Autodesk Inventor part; units mm, degrees
ref_plane "YZ Plane" through (0, 0, 0) normal (1, 0, 0) x (0, 1, 0)
ref_plane "XZ Plane" through (0, 0, 0) normal (0, 1, 0) x (-1, 0, 0)
ref_plane "XY Plane" through (0, 0, 0) normal (0, 0, 1) x (1, 0, 0)
sketch "Sketch1" plane through (0, 0, 0) normal (0, 1, 0) x (-1, 0, 0)
  line L0 (-19.65, 15.2) -> (19.65, 15.2)
  line L1 (19.65, 15.2) -> (19.65, -15.2)
  line L2 (19.65, -15.2) -> (-19.65, -15.2)
  line L3 (-19.65, -15.2) -> (-19.65, 15.2)
  line L4 (-19.65, 15.2) -> (19.65, -15.2) construction
  line L5 (19.65, 15.2) -> (-19.65, -15.2) construction
  point P0 (0, 0)
  dimension "d0" = 30.4
  dimension "d1" = 39.3
extrude "Extrusion1" add sketch "Sketch1" along normal blind 2
sketch "Sketch2" plane through (0, 0, 0) normal (0, -1, 0) x (1, 0, 0)
  circle A0 centre (-17.225, -12.775) radius 2.425
  circle A1 centre (-17.225, -12.775) radius 1.475
  line L0 (-19.65, -15.2) -> (19.65, -15.2)
  line L1 (-19.65, 15.2) -> (-19.65, -15.2)
  circle A2 centre (-17.225, 12.775) radius 1.475
  circle A3 centre (-17.225, 12.775) radius 2.425
  circle A4 centre (17.225, 12.775) radius 1.475
  circle A5 centre (17.225, 12.775) radius 2.425
  circle A6 centre (17.225, -12.775) radius 1.475
  circle A7 centre (17.225, -12.775) radius 2.425
  line L2 (19.65, 15.2) -> (-19.65, 15.2)
  line L3 (19.65, -15.2) -> (19.65, 15.2)
  point P0 (0, 0)
  dimension "d4" = 0.95
  dimension "d5" = 2.95
  dimension "d6" = 2.95
  dimension "d7" = 0.95
  dimension "d8" = 2.95
  dimension "d9" = 0.95
  dimension "d10" = 2.95
  dimension "d11" = 0.95
  dimension "d12" = 39.3
extrude "Extrusion3" add sketch "Sketch2" along normal blind 3.5 contours A0 | A3 | A7 | A5
sketch "Sketch3" plane through (0, 0, 0) normal (0, -1, 0) x (1, 0, 0)
  line L0 (-19.65, -15.2) -> (-17.225, -15.2)
  circle A0 centre (-17.225, 12.775) radius 2.425
  line L1 (-19.65, -15.2) -> (-18.15, -15.2)
  line L2 (-18.15, -15.2) -> (-18.15, 15.0167)
  line L3 (-18.15, 15.0167) -> (-19.65, 15.0167)
  line L4 (-19.65, 15.0167) -> (-19.65, -15.2)
  point P0 (0, 0)
  dimension "d17" = 1.5
extrude "Extrusion4" add sketch "Sketch3" along normal up to surface (3.5 mm away) contours L4 A0 L2 L0 | L4 L3 A0 | A0 L2 picked at (-18.7278, 13.0496)
sketch "Sketch4" plane through (0, 0, 0) normal (0, -1, 0) x (1, 0, 0)
  line L0 (19.65, -15.2) -> (-19.65, -15.2)
  line L1 (-19.65, -15.2) -> (-19.65, 15.2)
  line L2 (19.65, -15.2) -> (-19.65, -15.2)
  line L3 (-19.65, -15.2) -> (-19.65, -13.7)
  line L4 (-19.65, -13.7) -> (19.65, -13.7)
  line L5 (19.65, -13.7) -> (19.65, -15.2)
  point P0 (0, 0)
  dimension "d20" = 1.5
extrude "Extrusion5" add sketch "Sketch4" along normal up to surface (3.5 mm away)
sketch "Sketch5" plane through (0, 0, 0) normal (0, -1, 0) x (1, 0, 0)
  line L0 (-19.65, 15.0167) -> (-19.65, -15.2)
  line L1 (19.65, 15.2) -> (-19.65, 15.2)
  line L2 (-19.65, 15.2) -> (-19.65, 14)
  line L3 (-19.65, 14) -> (19.65, 14)
  line L4 (19.65, 14) -> (19.65, 15.2)
  point P0 (0, 0)
  dimension "d23" = 1.2
extrude "Extrusion6" add sketch "Sketch5" along normal up to surface (3.5 mm away)
sketch "Sketch6" plane through (0, 0, 0) normal (0, -1, 0) x (1, 0, 0)
  line L0 (-19.65, 15.2) -> (19.65, 15.2)
  line L1 (19.65, -15.2) -> (-19.65, -15.2)
  line L2 (19.65, 15.2) -> (18.45, 15.2)
  line L3 (18.45, 15.2) -> (18.45, -15.2)
  line L4 (18.45, -15.2) -> (19.65, -15.2)
  line L5 (19.65, -15.2) -> (19.65, 15.2)
  dimension "d27" = 1.2
extrude "Extrusion7" add sketch "Sketch6" along normal up to surface (3.5 mm away)
sketch "Sketch7" plane through (0, -3.5, 0) normal (0, -1, 0) x (1, 0, 0)
  arc A0 (16.4034, 14) -> (18.45, 11.9534) centre (17.225, 12.775) ccw
  circle A1 centre (17.225, 12.775) radius 1.475
  arc A2 (18.45, -11.9534) -> (16.0761, -13.7) centre (17.225, -12.775) ccw
  circle A3 centre (17.225, -12.775) radius 1.475
  arc A4 (-16.0761, -13.7) -> (-18.15, -11.6261) centre (-17.225, -12.775) ccw
  circle A5 centre (-17.225, -12.775) radius 1.475
  arc A6 (-18.15, 11.6261) -> (-16.4034, 14) centre (-17.225, 12.775) ccw
  circle A7 centre (-17.225, 12.775) radius 1.475
  point P0 (0, 0)
extrude "Extrusion8" cut sketch "Sketch7" against normal up to surface (5.5 mm away)
sketch "Sketch8" plane through (0, 2, 0) normal (0, 1, 0) x (1, 0, 0)
  line L0 (13.35, -7.2346) -> (-9.65, -7.2346)
  line L1 (-9.65, -7.2346) -> (-9.65, 8.7654)
  line L2 (-9.65, 8.7654) -> (13.35, 8.7654)
  line L3 (13.35, 8.7654) -> (13.35, -7.2346)
  line L4 (13.35, -7.2346) -> (-9.65, 8.7654) construction
  line L5 (-9.65, -7.2346) -> (13.35, 8.7654) construction
  line L6 (-19.65, 15.2) -> (-19.65, -15.2)
  point P0 (0, 0)
  point P1 (1.85, 0.7654)
  dimension "d34" = 23
  dimension "d35" = 10
  dimension "d40" = 16
extrude "Extrusion9" cut sketch "Sketch8" against normal up to surface (2 mm away)
chamfer "Chamfer1" distance 1 angle 45 4 edges at (-9.65, 0, -0.7654) (1.85, 0, 7.2346) (13.35, 0, -0.7654) (1.85, 0, -8.7654)
fillet "Fillet2" radius 1 4 edges at (-19.65, -0.75, 15.2) (19.65, -0.75, 15.2) (19.65, -0.75, -15.2) (-19.65, -0.75, -15.2)
fillet "Fillet3" radius 1.5 4 edges at (13.35, 1.5, -8.7654) (-9.65, 1.5, -8.7654) (-9.65, 1.5, 7.2346) (13.35, 1.5, 7.2346)
properties part number "Enclosure_Lid"
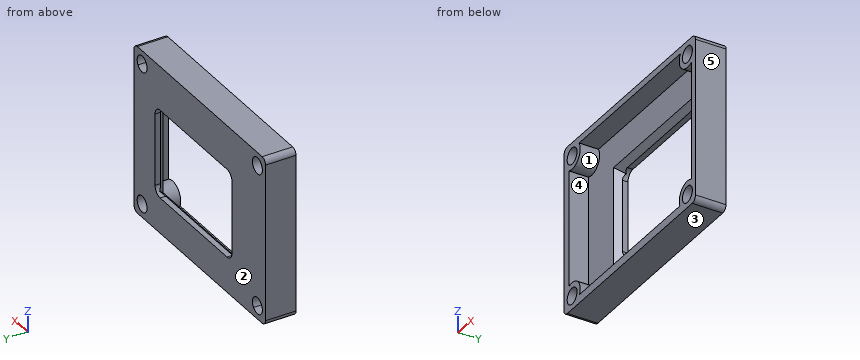
CAD build for the part. Positions are in the model's coordinates, mm. Face numbers are marked on the shaded views. A direction names the side the tool comes from. Round coordinates to 2 decimals unless told otherwise and drop trailing zeros. Order: outer loops, then holes, each group sorted by start corner. A loop starts at its lowest first (then second) coordinate and runs counter-clockwise, first axis right, second up. Notation, with made-up numbers: (-24.75, 55.25) -> (34.25, 55.25) arc R32 ccw to (34.25, 89.25) -> close; hole circle Ø9 at (-33.75, 80). An arc over 180 degrees is marked (long way). Write item = value, one per line. Start each with the question number.
(1) Cut at A-A, the plane z = -4. List the corners of the cut face in (x, y).
(2) Pull direction Z, two halves, no side cores. Call the marked faces 1, 2 and 3: released by +Z, released by -Z, zero draft, split by the parting line, or undercut.
(3) Which spindle directions (+Z, -Z, +X, -X, +Y, -Y) get a long thin tool onto all of the face, cutting with end or side? Do the marked faces 4 and 5. Say none if no direction does.
(4) Cut at B-B, the plane x = 6. List the corners of the cut face in (y, z), then the cut area to 4 significant figures.
(5) Cut at D-D, the plane z = 12.5. List the corners of the cut face in (x, y), then the cut area to 3 significant figures.
(6) Pin check, flat tips, straight feed: P1, Ø4, axis at x = -17.225, z = -12.775, coming from the -Y side; P2, Ø8, axis at x = -6.5, z = -1.5, coming from the -Y side; P3, Ø2.5, axis at x = 17.225, z = 12.775, coming from the -Y side. Stop position of each tip, or through.
(7) Cut at C-C, the plane y = -1.4. List the corners of the cut face in (x, z) (3 decimals), then the cut area to 3 significant figures.
(8) Probe line 1 (X direction, y = -2.9, z = 6.5); line 2 (Z direction, x = 13, y = -1.3); line 3 (Z direction, x = 17, y = 1.2). List the from-to ranges inside material, lowest first. Write a range as [from, to].
Model answer:
q1.outline = (-19.65, -3.5) -> (-18.15, -3.5) -> (-18.15, 0) -> (-10.65, 0) -> (-9.65, 1) -> (-9.65, 2) -> (-19.65, 2) -> close; (13.35, 1) -> (14.35, 0) -> (18.45, 0) -> (18.45, -3.5) -> (19.65, -3.5) -> (19.65, 2) -> (13.35, 2) -> close
q2.face_1 = undercut
q2.face_2 = zero draft
q2.face_3 = released by -Z
q3.face_4 = -Y
q3.face_5 = +Z, -Z, +X, +Y, -Y
q4.outline = (-3.5, -15.2) -> (2, -15.2) -> (2, -8.77) -> (1, -8.77) -> (0, -9.77) -> (0, -13.7) -> (-3.5, -13.7) -> close; (-3.5, 14) -> (0, 14) -> (0, 8.23) -> (1, 7.23) -> (2, 7.23) -> (2, 15.2) -> (-3.5, 15.2) -> close
q4.area = 37.25 mm2
q5.outline = (-19.65, -3.5) -> (-18.67, -3.5) -> (-18.67, 2) -> (-19.65, 2) -> close; (-15.78, -3.5) -> (-14.82, -3.5) -> (-14.82, 0) -> (14.82, 0) -> (14.82, -3.5) -> (15.78, -3.5) -> (15.78, 2) -> (-15.78, 2) -> close; (18.67, -3.5) -> (19.65, -3.5) -> (19.65, 2) -> (18.67, 2) -> close
q5.area = 80.6 mm2
q6.P1 = -3.5
q6.P2 = 0.15
q6.P3 = through
q7.outline = (-19.65, -14.2) arc R1 ccw to (-18.65, -15.2) -> (18.65, -15.2) arc R1 ccw to (19.65, -14.2) -> (19.65, 14.2) arc R1 ccw to (18.65, 15.2) -> (-18.65, 15.2) arc R1 ccw to (-19.65, 14.2) -> close; hole circle Ø2.95 at (-17.225, -12.775); hole circle Ø2.95 at (-17.225, 12.775); hole (-18.15, -10.533) arc R2.425 cw to (-14.983, -13.7) -> (14.983, -13.7) arc R2.425 cw to (18.45, -10.682) -> (18.45, 10.682) arc R2.425 cw to (15.132, 14) -> (-15.132, 14) arc R2.425 cw to (-18.15, 10.533) -> close; hole circle Ø2.95 at (17.225, -12.775); hole circle Ø2.95 at (17.225, 12.775)
q7.area = 196 mm2
q8.line_1 = [-19.65, -18.15], [18.45, 19.65]
q8.line_2 = [-15.2, -13.7], [14, 15.2]
q8.line_3 = [-15.2, -14.23], [-11.32, 11.32], [14.23, 15.2]
